```python
from build123d import *

# Parameters (mm, degrees)
SKETCH_W      = 100
SKETCH_H      = 12.5
PAD_DEPTH     = 60
SKETCH001_W   = 97.5
SKETCH001_H   = 2.5
POCKET_DEPTH  = 57.5
CHAMFER_SIZE2 = 90
CHAMFER_SIZE  = 50
FILLET_R      = 1


with BuildPart() as part:
    # Sketch (on XY_Plane of Origin) → Pad (new body)
    with BuildSketch(Plane.XY):
        Rectangle(SKETCH_W, SKETCH_H)
    extrude(amount=PAD_DEPTH)

    # Sketch001 (on Face6 of Pad) → Pocket (cut)
    with BuildSketch(Plane.XY.offset(60)):
        with Locations((-1.25, 2.5)):
            Rectangle(SKETCH001_W, SKETCH001_H)
        with Locations((-1.25, -2.5)):
            Rectangle(SKETCH001_W, SKETCH001_H)
    extrude(amount=-POCKET_DEPTH, mode=Mode.SUBTRACT)

    # Chamfer
    chamfer_edges = [part.edges().sort_by_distance(p)[0] for p in [
        (-50, 5, 60),
        (-50, 0, 60),
        (-50, -5, 60),
    ]]
    chamfer_side = part.faces().sort_by_distance((-50, 0, 29.222973))[0]
    chamfer(chamfer_edges, length=CHAMFER_SIZE, length2=CHAMFER_SIZE2, reference=chamfer_side)

    # Fillet
    fillet_edges = [part.edges().sort_by_distance(p)[0] for p in [
        (-50, -6.25, 5),
        (-50, -5, 10),
        (-50, 0, 0),
        (-50, -3.75, 6.25),
        (-50, 6.25, 5),
        (-50, -2.5, 2.5),
        (-50, 5, 10),
        (-50, -1.25, 6.25),
        (-50, 3.75, 6.25),
        (-50, 0, 10),
        (-50, 2.5, 2.5),
        (-50, 1.25, 6.25),
        (-5, -6.25, 35),
        (0, -6.25, 0),
        (45, -6.25, 60),
        (50, -6.25, 30),
        (-5, -3.75, 35),
        (40, -5, 60),
        (50, 0, 0),
        (0, 6.25, 0),
        (-1.25, -3.75, 2.5),
        (43.75, -3.75, 60),
        (47.5, -3.75, 31.25),
        (-5, 6.25, 35),
        (45, 6.25, 60),
        (50, 6.25, 30),
        (47.5, -2.5, 2.5),
        (-1.25, -1.25, 2.5),
        (40, 5, 60),
        (-5, 3.75, 35),
        (-5, -1.25, 35),
        (43.75, -1.25, 60),
        (47.5, -1.25, 31.25),
        (-1.25, 3.75, 2.5),
        (43.75, 3.75, 60),
        (47.5, 3.75, 31.25),
        (-5, 1.25, 35),
        (40, 0, 60),
        (-1.25, 1.25, 2.5),
        (47.5, 2.5, 2.5),
        (43.75, 1.25, 60),
        (47.5, 1.25, 31.25),
        (50, 0, 60),
        (47.5, 2.5, 60),
        (47.5, -2.5, 60),
    ]]
    fillet(fillet_edges, radius=FILLET_R)


solid = part.part
```
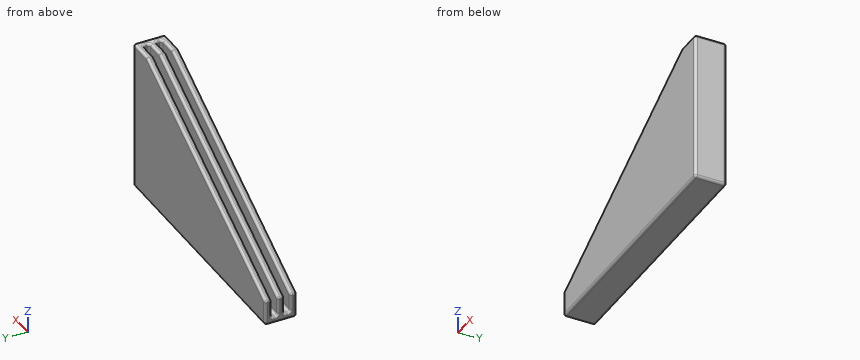
Check sheet for the modelled part. Datum: model origin and axes. Units: mm. Coordinates: 2 decimals unless noted, no trailing zeros. Loops run counter-clockwise (first coordinate to the right, second up) from the corner with the lowest first, then second, coordinate; pieces in that order, holes last.
1) Sectioned sample at A-A (z = 5.5). Record the boundary of the cut face in (x, y).
2) Material ranges on probe 1 along Y at (x, z) = (41.5, 26.5); probe 2 along X at (y, z) = (2.25, 20); probe 3 along Z at (x, y) = (33.5, -2.75), recorded low to high.
3) Gauge pin test, flat ends, axial feed: pin 1 (0.6 mm diameter, centred on x = 14, y = -2.5, fed in from +Z); pin 2 (2 mm diameter, centred on x = -7.5, y = -3.5, fed in from +Z). Record the tip position at first contact, or that the pin passes through.
Check sheet entries:
1. outline: (-50, -5.25) arc R1 ccw to (-49, -6.25) - (49, -6.25) arc R1 ccw to (50, -5.25) - (50, 5.25) arc R1 ccw to (49, 6.25) - (-49, 6.25) arc R1 ccw to (-50, 5.25) - (-50, 4.75) arc R1 ccw to (-49, 3.75) - (46.5, 3.75) arc R1 cw to (47.5, 2.75) - (47.5, 2.25) arc R1 cw to (46.5, 1.25) - (-49, 1.25) arc R1 ccw to (-50, 0.25) - (-50, -0.25) arc R1 ccw to (-49, -1.25) - (46.5, -1.25) arc R1 cw to (47.5, -2.25) - (47.5, -2.75) arc R1 cw to (46.5, -3.75) - (-49, -3.75) arc R1 ccw to (-50, -4.75) - close
2. probe 1: y = -6.25 to -3.75, -1.25 to 1.25, 3.75 to 6.25
2. probe 2: x = 47.5 to 50
2. probe 3: z = 0 to 2.5
3. pin 1: stops at z = 2.5
3. pin 2: stops at z = 33.83
